Verification items for the finished model (mm, model axes). Give positions to 0.01 mm unless a question says otherwise; leave off trailing zeros. Order: outer loops, then holes, each group sorted by start corner. A loop starts at its lowest first (then second) coordinate and runs counter-clockwise, first axis right, second up.
from build123d import *

# Parameters (mm, degrees)
F0_W        = 114.3
F0_H        = 10
F1_DEPTH    = 2
F2_R        = 5.08
F3_R        = 5.08
F4_T1_DEPTH = 27.3873984488
F5_T1_DEPTH = 27.3873984488


# Not quite as in the source:
# - a fillet or chamfer that OpenCascade refuses, or shapes differently, is made with other operations: its cross-section is extruded or revolved along the edge and cut away or added


with BuildPart() as f1:
    # F0 (on Top) → F1 (new body)
    with BuildSketch(Plane.XY):
        with Locations((-2.3567027405, -37.438484022)):
            Rectangle(F0_W, F0_H)
    extrude(amount=F1_DEPTH)

    # F2
    f2_edges = [f1.edges().sort_by_distance(p)[0] for p in [
        (-59.506703, -32.438484, 1),
    ]]
    fillet(f2_edges, radius=F2_R)

    # F3
    f3_edges = [f1.edges().sort_by_distance(p)[0] for p in [
        (54.793297, -32.438484, 1),
    ]]
    fillet(f3_edges, radius=F3_R)

    # F4: fillet of radius 5.08 on 1 edges, made by hand

    # F4_s2 → F4_t1 (cut)
    with BuildSketch(Plane.XY.offset(-12.6936992244)):
        with BuildLine():
            ThreePointArc((-59.5067027405, -37.518484022), (-57.9643043793, -41.0067164708), (-54.4292230507, -42.438484022))
            Line((-54.4292230507, -42.438484022), (-59.5067027405, -42.438484022))
            Line((-59.5067027405, -42.438484022), (-59.5067027405, -37.518484022))
        make_face()
    extrude(amount=F4_T1_DEPTH, mode=Mode.SUBTRACT)

    # F5: fillet of radius 5.08 on 1 edges, made by hand

    # F5_s2 → F5_t1 (cut)
    with BuildSketch(Plane.XY.offset(-12.6936992244)):
        with BuildLine():
            ThreePointArc((54.7932972595, -37.518484022), (53.2508988984, -41.0067164708), (49.7158175697, -42.438484022))
            Line((49.7158175697, -42.438484022), (54.7932972595, -42.438484022))
            Line((54.7932972595, -42.438484022), (54.7932972595, -37.518484022))
        make_face()
    extrude(amount=F5_T1_DEPTH, mode=Mode.SUBTRACT)


solid = f1.part
(1) Scan lines: line 1 (Y direction, x = 50, z = 1.3); line 2 (X direction, y = -33.5, z = 1.6); line 3 (X direction, y = -39, z = 0.7). Record each from-to range of solid material in increasing order.
Solved:
line 1: y = -42.43 to -32.45
line 2: x = -57.53 to 52.82
line 3: x = -59.24 to 54.52
(2) Section check C-C, the plane y = -41. Enter the section's corners in (x, z).
Solved:
outline: (-57.97, 0) - (53.26, 0) - (53.26, 2) - (-57.97, 2) - close
(3) Section check B-B, the plane y = -34.5. Enter the section's corners in (x, z).
Solved:
outline: (-58.51, 0) - (53.8, 0) - (53.8, 2) - (-58.51, 2) - close
(4) Section check A-A, the plane z = 1.7. Enter the section's corners in (x, y).
Solved:
outline: (-59.51, -37.52) arc R5.08 ccw to (-54.43, -42.44) - (49.72, -42.44) arc R5.08 ccw to (54.79, -37.52) arc R5.08 ccw to (49.71, -32.44) - (-54.43, -32.44) arc R5.08 ccw to start
